Check sheet for the modelled part. Datum: model origin and axes. Units: mm. A direction names the side the tool comes from. Round coordinates to 2 decimals unless told otherwise and drop trailing zeros. Write each loop counter-clockwise with the first axis right and the second up, starting at its lowest first coordinate (ties: lowest second). Pieces come first, ordered by that corner, then holes. Notation, with made-up numbers: (-28.5, 60) -> (-16.5, 60) arc R9 ccw to (-16.5, 77) -> close; hole circle Ø10 at (-8.5, 35). An arc over 180 degrees is marked (long way). One line per item, written item: value. Start each with the question number.
```python
from build123d import *

# Parameters (mm, degrees)
BOSS_EXTRUDE1_DEPTH = 50
FILLET1_R           = 15


with BuildPart() as part:
    # Sketch1 → Boss-Extrude1 (new body)
    with BuildSketch(Plane.XY):
        Polygon((-37.5, -200), (-37.5, 0), (37.5, 0), (37.5, -200), (77.5, -200), (77.5, 50), (-77.5, 50), (-77.5, -200), align=None)
    extrude(amount=BOSS_EXTRUDE1_DEPTH)

    # Fillet1
    fillet1_edges = [part.edges().sort_by_distance(p)[0] for p in [
        (-57.5, -200, 0),
        (-77.5, -200, 25),
        (-77.5, 50, 25),
        (77.5, 50, 25),
        (77.5, -200, 25),
        (57.5, -200, 50),
        (77.5, -75, 50),
        (0, 50, 50),
        (-77.5, -75, 50),
        (-57.5, -200, 50),
        (-77.5, -75, 0),
        (0, 50, 0),
        (77.5, -75, 0),
        (57.5, -200, 0),
    ]]
    fillet(fillet1_edges, radius=FILLET1_R)


solid = part.part
```
1. Material ranges on probe 1 along X at (y, z) = (-75, 21.5); probe 2 along Y at (x, z) = (-10.5, 20.5); probe 3 along X at (y, z) = (-86.5, 46), recorded low to high.
2. Cross-section at B-B (z = 18.5). Record the cut outline in (x, y).
3. Access from +Z, -Z, +X, -X, +Y, -Y to the whole of each face (thin tool, end or side, straight path). Record for faces 1 (the face through (1, 50, 25)), 2 (the face through (-1, 0, 25)).
4. Depth check by flat-ended pin: pin 1 Ø2 at (y, z) = (-154.5, 36.5) entering from +X; pin 2 Ø1.5 at (x, z) = (-17, 35) entering from -Y; pin 3 Ø10 at (x, z) = (38.5, 45) entering from +Y. Enter the tip coordinate at first touch or a pass-through.
5. Release check for a two-part mould opening along X. For faces 3 (the face through (-49.82, -195.72, 4.51)), 4 (the face through (-37.5, -101, 25)), 5 (the face through (-73.22, -76.54, 4.51)), 6 (the face through (37.5, -99, 25)) record: +X half, -X half, draft (parallel to the pull), parting line (faces both ways), or undercut.
6. Cross-section at C-C (x = -47.5). Record the cut outline in (y, z), plus the area to 3 significant figures.
7. Cross-section at D-D (z = 4). Record the cut outline in (x, y), plus the area to 3 significant figures.
8. Cross-section at A-A (y = -26). Record the cut outline in (x, z), plus the area to 3 significant figures.
Working result:
1. probe 1: x = -77.5 to -37.5, 37.5 to 77.5
1. probe 2: y = 0 to 50
1. probe 3: x = -72.7 to -37.5, 37.5 to 72.7
2. outline: (-77.5, -185) arc R15 ccw to (-62.5, -200) -> (-37.5, -200) -> (-37.5, 0) -> (37.5, 0) -> (37.5, -200) -> (62.5, -200) arc R15 ccw to (77.5, -185) -> (77.5, 35) arc R15 ccw to (62.5, 50) -> (-62.5, 50) arc R15 ccw to (-77.5, 35) -> close
3. face 1: +Z, -Z, +X, -X, +Y
3. face 2: +Z, -Z, -Y
4. pin 1: stops at x = 77.49
4. pin 2: stops at y = 0
4. pin 3: stops at y = 49.14
5. face 3: draft
5. face 4: undercut
5. face 5: -X half
5. face 6: undercut
6. outline: (-200, 15) arc R15 ccw to (-185, 0) -> (35, 0) arc R15 ccw to (50, 15) -> (50, 35) arc R15 ccw to (35, 50) -> (-185, 50) arc R15 ccw to (-200, 35) -> close
6. area: 12,300 mm^2
7. outline: (-72.7, -185) arc R10.2 ccw to (-62.5, -195.2) -> (-37.5, -195.2) -> (-37.5, 0) -> (37.5, 0) -> (37.5, -195.2) -> (62.5, -195.2) arc R10.2 ccw to (72.7, -185) -> (72.7, 35) arc R10.2 ccw to (62.5, 45.2) -> (-62.5, 45.2) arc R10.2 ccw to (-72.7, 35) -> close
7. area: 20,200 mm^2
8. outline: (-77.5, 15) arc R15 ccw to (-62.5, 0) -> (-37.5, 0) -> (-37.5, 50) -> (-62.5, 50) arc R15 ccw to (-77.5, 35) -> close; (37.5, 0) -> (62.5, 0) arc R15 ccw to (77.5, 15) -> (77.5, 35) arc R15 ccw to (62.5, 50) -> (37.5, 50) -> close
8. area: 3,810 mm^2
